Model file for the job. Use its own axes, mm. Round coordinates to 2 decimals unless told otherwise and drop trailing zeros. Write each loop counter-clockwise with the first axis right and the second up, starting at its lowest first coordinate (ties: lowest second). Pieces come first, ordered by that corner, then holes. Notation, with made-up numbers: (17, 80) - (75, 80) arc R12 ccw to (75, 91) - close; hole circle Ø8 at (-25.75, -3.75). An arc over 180 degrees is marked (long way). Answer as a JSON object with one key per item and string values. Group by question number.
from build123d import *

# Parameters (mm, degrees)
SKETCH1_W           = 127
SKETCH1_H           = 95.25
BOSS_EXTRUDE1_DEPTH = 3.175
SKETCH2_W           = 25.4
SKETCH2_H           = 3.175
BOSS_EXTRUDE2_DEPTH = 3.175
SKETCH3_W           = 25.4
SKETCH3_H           = 3.175
BOSS_EXTRUDE3_DEPTH = 3.175
SKETCH4_W           = 25.4
SKETCH4_H           = 3.175
BOSS_EXTRUDE4_DEPTH = 3.175
SKETCH5_W           = 25.4
SKETCH5_H           = 3.175
BOSS_EXTRUDE5_DEPTH = 3.175


with BuildPart() as part:
    # Sketch1 → Boss-Extrude1 (new body)
    with BuildSketch(Plane(origin=(0, 0, 0), x_dir=(1, 0, 0), z_dir=(0, 1, 0))):
        with Locations((64.375862069, 2.737068966)):
            Rectangle(SKETCH1_W, SKETCH1_H)
    extrude(amount=BOSS_EXTRUDE1_DEPTH)

    # Sketch2 → Boss-Extrude2 (add)
    with BuildSketch(Plane(origin=(127.875862069, 0, 0), x_dir=(0, 0, -1), z_dir=(1, 0, 0))):
        with Locations((2.737068966, 1.5875)):
            Rectangle(SKETCH2_W, SKETCH2_H)
    extrude(amount=BOSS_EXTRUDE2_DEPTH)

    # Sketch3 → Boss-Extrude3 (add)
    with BuildSketch(Plane.ZY.offset(-0.875862069)):
        with Locations((-2.737068966, 1.5875)):
            Rectangle(SKETCH3_W, SKETCH3_H)
    extrude(amount=BOSS_EXTRUDE3_DEPTH)

    # Sketch4 → Boss-Extrude4 (add)
    with BuildSketch(Plane(origin=(0, 0, -50.362068966), x_dir=(-1, 0, 0), z_dir=(0, 0, -1))):
        with Locations((-64.375862069, 1.5875)):
            Rectangle(SKETCH4_W, SKETCH4_H)
    extrude(amount=BOSS_EXTRUDE4_DEPTH)

    # Sketch5 → Boss-Extrude5 (add)
    with BuildSketch(Plane.XY.offset(44.887931034)):
        with Locations((64.375862069, 1.5875)):
            Rectangle(SKETCH5_W, SKETCH5_H)
    extrude(amount=BOSS_EXTRUDE5_DEPTH)


solid = part.part
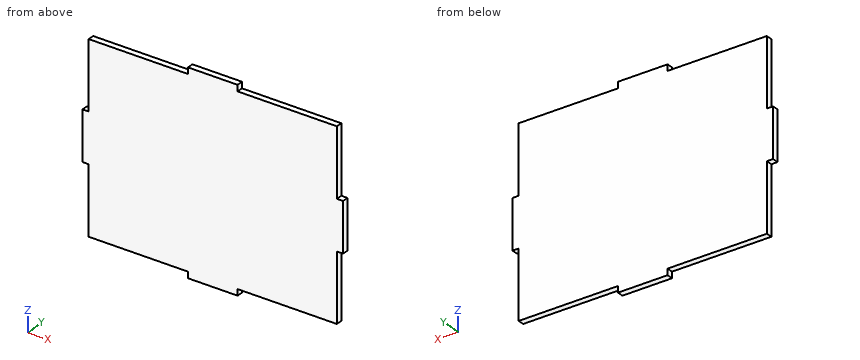
(1) Drill centre lines: line 1 (Z direction, x = 15, y = 2.25); line 2 (X direction, y = 1.55, z = -26). Where is each one in solid material? Low to high. Write a range as from..to.
(2) Slice it at A-A (y = 0.95). Write the cut outline in (x, z).
(3) Flat gauge pins, fed straight in: pin 1 (1 mm diameter, centred on y = 2, z = -33, fed in from +X); pin 2 (1 mm diameter, centred on x = 13.5, y = 1.5, fed in from -Z); pin 3 (1.6 mm diameter, centred on x = 108.5, y = 1.5, fed in from +Z). Where does each tip first touch, or does it go through?
(4) Slice it at B-B (z = 21). Write the cut outline in (x, y) (3 decimals).
(5) Slice it at C-C (x = 30.5). Write the cut outline in (y, z) (3 decimals).
Answer:
{
 "1": {"line 1": "-50.36..44.89", "line 2": "0.88..127.88"},
 "2": {"outline": "(-2.3, -15.44) - (0.88, -15.44) - (0.88, -50.36) - (51.68, -50.36) - (51.68, -53.54) - (77.08, -53.54) - (77.08, -50.36) - (127.88, -50.36) - (127.88, -15.44) - (131.05, -15.44) - (131.05, 9.96) - (127.88, 9.96) - (127.88, 44.89) - (77.08, 44.89) - (77.08, 48.06) - (51.68, 48.06) - (51.68, 44.89) - (0.88, 44.89) - (0.88, 9.96) - (-2.3, 9.96) - close"},
 "3": {"pin 1": "x = 127.88", "pin 2": "z = -50.36", "pin 3": "z = 44.89"},
 "4": {"outline": "(0.876, 0) - (127.876, 0) - (127.876, 3.175) - (0.876, 3.175) - close"},
 "5": {"outline": "(0, -50.362) - (3.175, -50.362) - (3.175, 44.888) - (0, 44.888) - close"}
}
